Geometry: final body of the model. Coordinates: model frame, mm. Face numbers are marked on the shaded views. A direction names the side the tool comes from. Coordinates: 2 decimals unless noted, no trailing zeros. Order: outer loops, then holes, each group sorted by start corner. A loop starts at its lowest first (then second) coordinate and runs counter-clockwise, first axis right, second up. Notation, with made-up numbers: (9, 55) - (53, 55) arc R31 ccw to (53, 90) - close; hole circle Ø6 at (38, 2.5). An arc over 180 degrees is marked (long way). Use a Markdown table: item, result. Add a question column.
```python
from build123d import *

# Parameters (mm, degrees)
SKETCH1_R                = 2.5
BOSS_EXTRUDE1_DEPTH      = 15
FILLET4_R                = 2
SKETCH9_W                = 5
SKETCH9_H                = 12
CUT_EXTRUDE1_DEPTH       = 13.0000001
CUT_EXTRUDE1_DEPTH_BACK  = 13.0000001
SKETCH10_R               = 5
BOSS_EXTRUDE2_DEPTH      = 22.5
BOSS_EXTRUDE2_DEPTH_BACK = 7.5


with BuildPart() as part:
    # Sketch1 → Boss-Extrude1 (new body)
    with BuildSketch(Plane.XY):
        with BuildLine():
            ThreePointArc((7.868400372, 78.554913295), (0, 88), (-7.868400372, 78.554913295))
            ThreePointArc((-7.868400372, 78.554913295), (-5.349774026, 40.71787649), (-11.535875122, 3.305084746))
            ThreePointArc((-11.535875122, 3.305084746), (0, -12), (11.535875122, 3.305084746))
            ThreePointArc((11.535875122, 3.305084746), (5.349774026, 40.71787649), (7.868400372, 78.554913295))
        make_face()
        with Locations((0, 80)):
            Circle(SKETCH1_R, mode=Mode.SUBTRACT)
    extrude(amount=BOSS_EXTRUDE1_DEPTH)

    # Fillet4
    fillet4_edges = [part.edges().sort_by_distance(p)[0] for p in [
        (5.349774026, 40.71787649, 15),
        (0, 88, 15),
        (-5.349774026, 40.71787649, 15),
        (0, 88, 0),
        (5.349774026, 40.71787649, 0),
        (0, -12, 0),
        (-5.349774026, 40.71787649, 0),
        (0, -12, 15),
    ]]
    fillet(fillet4_edges, radius=FILLET4_R)

    # Sketch9 → Cut-Extrude1 (cut, two sides)
    with BuildSketch(Plane(origin=(0, 0, 0), x_dir=(0, 0, -1), z_dir=(1, 0, 0))) as cut_extrude1_sk:
        with Locations((-7.5, 82.000003295)):
            Rectangle(SKETCH9_W, SKETCH9_H)
    extrude(amount=CUT_EXTRUDE1_DEPTH, mode=Mode.SUBTRACT)
    extrude(cut_extrude1_sk.sketch, amount=-CUT_EXTRUDE1_DEPTH_BACK, mode=Mode.SUBTRACT)

    # Sketch10 → Boss-Extrude2 (add, two sides)
    with BuildSketch(Plane.XY) as boss_extrude2_sk:
        Circle(SKETCH10_R)
    extrude(amount=BOSS_EXTRUDE2_DEPTH)
    extrude(boss_extrude2_sk.sketch, amount=-BOSS_EXTRUDE2_DEPTH_BACK)


solid = part.part
```
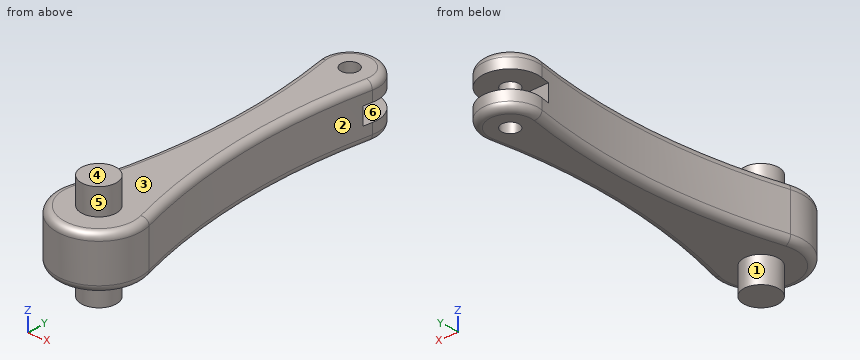
1) Set-up query: the marked faces 4, 5 and 6. Return all of +Z, -Z, +X, -X, +Y, -Y with unobstructed straight access to the full face (end or side cutting, diameter ignored); none if empty.
2) Ray query, line 1 along X through (y, z) = (80, 2.7); line 2 along Z through (x, y) = (-2.25, 75.5); line 3 along Z through (x, y) = (-7, 82). Return the intervals inside material, ascending.
3) Section A-A (x = 0). Return loops of the section in (y, z), then the cut area to 3 significant figures.
4) Section B-B (y = 80). Give the number of separate pieces and of enclosed holes in the cut face, then the cut area to 3 significant figures.
5) Draft query along Y for the marked faces 1, 2 and 3. Return one class per face: pulls with the +Y half, pulls with the -Y half, needs draft (parallel to the pull), parting line crosses it, or undercut.
6) Pin query (flat end, axial travel): pin 1 (2 mm diameter, centred on y = 37, z = 11, fed in from +X); pin 2 (2.5 mm diameter, centred on x = 0.5, z = 7.5, fed in from +Y); pin 3 (2 mm diameter, centred on x = 0, y = 17, fed in from +Z). Return the tip coordinate at first contact, or that it passes through.
7) Section C-C (z = 7). Return loops of the section in (x, y).
Values follow:
| question | item | result |
|---|---|---|
| 1 | face 4 | +Z, +X, -X, +Y, -Y |
| 1 | face 5 | +Z |
| 1 | face 6 | +X, -X, +Y |
| 2 | line 1 | x = -8 to -2.5, 2.5 to 8 |
| 2 | line 2 | z = 0 to 15 |
| 2 | line 3 | z = 0.46 to 5, 10 to 14.54 |
| 3 | outline | (-12, 2) arc R2 ccw to (-10, 0) - (-5, 0) - (-5, -7.5) - (5, -7.5) - (5, 0) - (77.5, 0) - (77.5, 5) - (76, 5) - (76, 10) - (77.5, 10) - (77.5, 15) - (5, 15) - (5, 22.5) - (-5, 22.5) - (-5, 15) - (-10, 15) arc R2 ccw to (-12, 13) - close; (82.5, 0) - (86, 0) arc R2 ccw to (88, 2) - (88, 5) - (82.5, 5) - close; (82.5, 10) - (88, 10) - (88, 13) arc R2 ccw to (86, 15) - (82.5, 15) - close |
| 3 | area | 1,540 mm² |
| 4 | separate pieces | 4 |
| 4 | enclosed holes | 0 |
| 4 | area | 107 mm² |
| 5 | face 1 | parting line crosses it |
| 5 | face 2 | undercut |
| 5 | face 3 | needs draft |
| 6 | pin 1 | stops at x = 5.65 |
| 6 | pin 2 | stops at y = 76 |
| 6 | pin 3 | stops at z = 15 |
| 7 | outline | (-11.54, 3.31) arc R12 ccw (long way) to (11.54, 3.31) arc R165 cw to (7.42, 76) - (-7.42, 76) arc R165 cw to start |
